Part print with two shaded views. Sizes in mm from the minimum x, y, z corner. A direction names the side the tool comes from. Round coordinates to 2 decimals unless told otherwise and drop trailing zeros. Order: outer loops, then holes, each group sorted by start corner. A loop starts at its lowest first (then second) coordinate and runs counter-clockwise, first axis right, second up. Notation, with made-up numbers: (86.25, -33) - (145.25, -33) arc R4 ccw to (145.25, -27) - close; hole circle Ø11 at (-40, 41.25). An arc over 180 degrees is marked (long way). Write item = value, one per line.
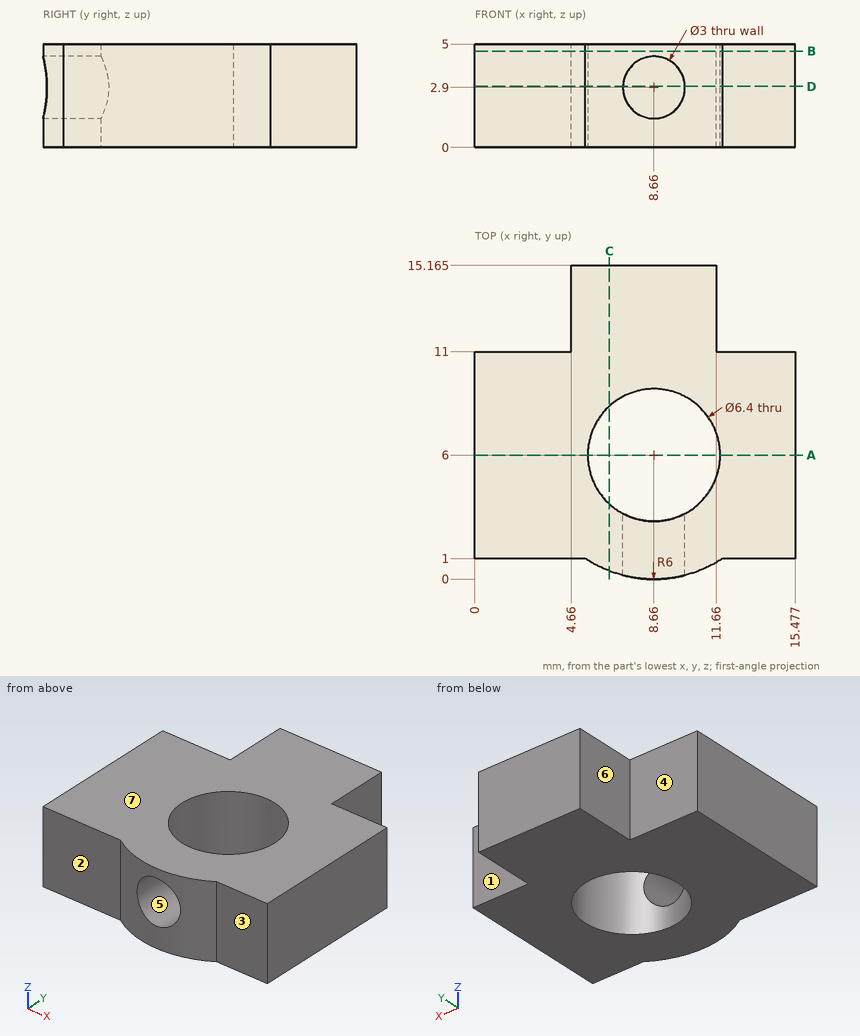
1) 3-axis set-ups, long thin cutter, end or side, ignore diameter. For the marked faces 1, 2, 3 and 4: which of +Z, -Z, +X, -X, +Y, -Y reach the whole face in a straight line?
Conclusion:
face_1 = +Z, -Z, +X, +Y
face_2 = +Z, -Z, -X, -Y
face_3 = +Z, -Z, +X, -Y
face_4 = +Z, -Z, -X, +Y
2) Cut at D-D (z = 2.95). Write the cut outline in (x, y) (1 decimal).
Conclusion:
outline = (0, 1) - (5.3, 1) arc R6 ccw to (7.2, 0.2) - (7.2, 3.2) arc R3.2 cw (long way) to (10.2, 3.2) - (10.2, 0.2) arc R6 ccw to (12, 1) - (15.5, 1) - (15.5, 11) - (11.7, 11) - (11.7, 15.2) - (4.7, 15.2) - (4.7, 11) - (0, 11) - close
3) Mould opens along X. For the marked faces 5, 6 and 7 say: +X half, -X half, draft (parallel to the pull), parting line (faces both ways), or undercut.
Conclusion:
face_5 = undercut
face_6 = -X half
face_7 = draft
4) Flat gauge pins, fed straight in: pin 1 Ø2.5 at (x, z) = (3.5, 1.5) entering from -Y; pin 2 Ø2 at (y, z) = (13, 3) entering from +X; pin 3 Ø1.2 at (y, z) = (13, 3.5) entering from -X. Where does each tip first touch, or does it go through?
Conclusion:
pin_1 = 1
pin_2 = 11.66
pin_3 = 4.66
5) Wall check: line 1 along X through (y, z) = (2.35, 2.9); line 2 along Y through (x, z) = (4.5, 2.8); line 3 along Y through (x, z) = (10, 2.1) (1 decimal). Give the ranges that are in metal, low to high.
Conclusion:
line_1 = 0 to 7.16, 10.16 to 15.48
line_2 = 1 to 11
line_3 = 0.2 to 3.1, 8.9 to 15.2
6) Cut at B-B (z = 4.65). Write the cut outline in (x, y) (1 decimal), and give its area (3 significant figures).
Conclusion:
outline = (0, 1) - (5.3, 1) arc R6 ccw to (12, 1) - (15.5, 1) - (15.5, 11) - (11.7, 11) - (11.7, 15.2) - (4.7, 15.2) - (4.7, 11) - (0, 11) - close; hole circle Ø6.4 at (8.7, 6)
area = 156 mm^2
7) Cut at A-A (y = 6). Write the cut outline in (x, z), and give its area (3 significant figures).
Conclusion:
outline = (0, 0) - (5.46, 0) - (5.46, 5) - (0, 5) - close; (11.86, 0) - (15.48, 0) - (15.48, 5) - (11.86, 5) - close
area = 45.4 mm^2
8) Cut at C-C (x = 6.5). Write the cut outline in (y, z) (1 decimal).
Conclusion:
outline = (0.4, 0) - (3.6, 0) - (3.6, 5) - (0.4, 5) - close; (8.4, 0) - (15.2, 0) - (15.2, 5) - (8.4, 5) - close
